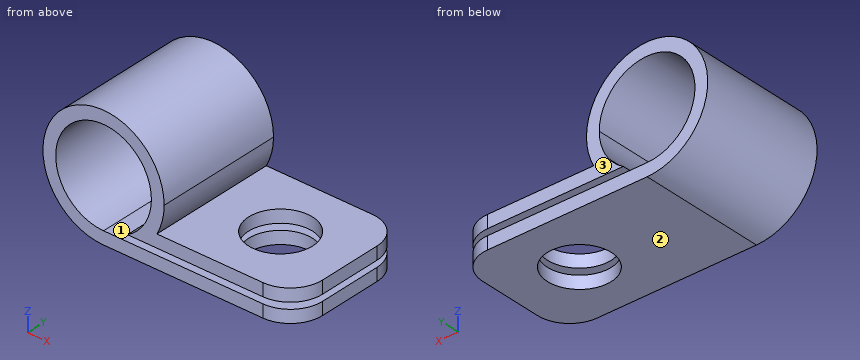
from build123d import *

# Parameters (mm, degrees)
F1_DEPTH = 8
F2_R     = 2
F3_DEPTH = 25
F4_R     = 2


# Not quite as in the source:
# - a feature names something its author has since deleted; it is built from what else it names


with BuildPart() as f1:
    # F0 (on Front) → F1 (new body)
    with BuildSketch(Plane.XZ):
        with BuildLine():
            ThreePointArc((0, -3), (-2.1213203436, 2.1213203436), (3, 0))
            ThreePointArc((3, 0), (2.8460498942, -0.9486832981), (2.4, -1.8))
            Line((2.4, -1.8), (3.3466401061, -1.8))
            ThreePointArc((3.3466401061, -1.8), (3.6849173941, -0.9281076437), (3.8, 0))
            ThreePointArc((3.8, 0), (-2.6870057685, 2.6870057685), (0, -3.8))
            Line((0, -3.8), (0, -3))
        make_face()
        with BuildLine():
            Line((2.3323807579, -3), (0, -3))
            Line((0, -3), (0, -3.8))
            ThreePointArc((0, -3.8), (1.2328828006, -3.5944401511), (2.3323807579, -3))
        make_face()
        with BuildLine():
            Line((3.3466401061, -1.8), (2.4, -1.8))
            ThreePointArc((2.4, -1.8), (1.9889684627, -2.2458861178), (1.4966629547, -2.6))
            Line((1.4966629547, -2.6), (2.7712812921, -2.6))
            ThreePointArc((2.7712812921, -2.6), (3.0850025217, -2.2187292402), (3.3466401061, -1.8))
        make_face()
        with BuildLine():
            Line((12, -3), (2.3323807579, -3))
            ThreePointArc((2.3323807579, -3), (1.2328828006, -3.5944401511), (0, -3.8))
            Line((0, -3.8), (12, -3.8))
            Line((12, -3.8), (12, -3))
        make_face()
        with BuildLine():
            Line((12, -1.8), (3.3466401061, -1.8))
            ThreePointArc((3.3466401061, -1.8), (3.0850025217, -2.2187292402), (2.7712812921, -2.6))
            Line((2.7712812921, -2.6), (12, -2.6))
            Line((12, -2.6), (12, -1.8))
        make_face()
    extrude(amount=F1_DEPTH)

    # F2 (on face) → F3 (cut)
    with BuildSketch(Plane.XY.offset(-1.8)):
        with Locations((7.6733200531, -4)):
            Circle(F2_R)
    extrude(amount=-F3_DEPTH, mode=Mode.SUBTRACT)

    # F4
    f4_edges = [f1.edges().sort_by_distance(p)[0] for p in [
        (12, -8, -2.2),
        (12, -8, -3.4),
        (12, 0, -3.4),
        (12, 0, -2.2),
    ]]
    fillet(f4_edges, radius=F4_R)


solid = f1.part
Design review of the part built by this model. Coordinates are the model's own, in mm. Face numbers are marked on the shaded views. Coordinates: 2 decimals unless noted, no trailing zeros. Order: outer loops, then holes, each group sorted by start corner. A loop starts at its lowest first (then second) coordinate and runs counter-clockwise, first axis right, second up. Notation, with made-up numbers: M 56,-13 L 80,-13 A10 cw 80,5 Z; hole C 28.5,39.5 d10. An arc over 180 degrees is marked long. Use a Markdown table: item, result.
(1) Add section A-A (y = -5.25). Give the boundary of the cut face in (x, z).
Worked answers:
| item | result |
|---|---|
| outline | M 0,-3.8 L 6.11,-3.8 L 6.11,-3 L 0,-3 A3 cw long 1.5,-2.6 L 6.11,-2.6 L 6.11,-1.8 L 3.35,-1.8 A3.8 ccw long Z; M 9.23,-3.8 L 12,-3.8 L 12,-3 L 9.23,-3 Z; M 9.23,-2.6 L 12,-2.6 L 12,-1.8 L 9.23,-1.8 Z |
(2) Add section C-C (z = -2). Give the boundary of the cut face in (x, y), then the cut area to 3 significant figures.
Worked answers:
| item | result |
|---|---|
| outline | M -3.23,-8 L -2.24,-8 L -2.24,0 L -3.23,0 Z; M 2.24,-8 L 10,-8 A2 ccw 12,-6 L 12,-2 A2 ccw 10,0 L 2.24,0 Z; hole C 7.67,-4 d4 |
| area | 71.8 mm2 |
(3) Wall thickness on probe 1 along X at (y, z) = (-6, 0); probe 2 along Z at (x, y) = (1.75, -2.5): over which ranges is each line inside the solid? List them lowest first.
Worked answers:
| item | result |
|---|---|
| probe 1 | x = -3.8 to -3, 3 to 3.8 |
| probe 2 | z = -3.8 to -3, -2.6 to -2.44, 2.44 to 3.37 |
(4) Add section D-D (z = 2.5). Give the boundary of the cut face in (x, y).
Worked answers:
| item | result |
|---|---|
| outline | M -2.86,-8 L -1.66,-8 L -1.66,0 L -2.86,0 Z; M 1.66,-8 L 2.86,-8 L 2.86,0 L 1.66,0 Z |
(5) For P1, Ø2.5, axis at x = 6.5, y = -4, coming from the +Z side, flat-tipped, find the tip position at first contact; note if it passes through.
Worked answers:
| item | result |
|---|---|
| P1 | stops at z = -1.8 |
(6) Draft analysis for pull direction Z (two halves, no side actions). For the marked faces 1, 2 and 3, state which applies: released by +Z, released by -Z, zero draft, split by the parting line, or undercut.
Worked answers:
| item | result |
|---|---|
| face 1 | undercut |
| face 2 | released by -Z |
| face 3 | zero draft |
(7) Add section B-B (x = 1). Give the boundary of the cut face in (y, z), then the cut area to 3 significant figures.
Worked answers:
| item | result |
|---|---|
| outline | M -8,-3.8 L 0,-3.8 L 0,-3 L -8,-3 Z; M -8,2.83 L 0,2.83 L 0,3.67 L -8,3.67 Z |
| area | 13.1 mm2 |
